```python
from build123d import *

# Parameters (mm, degrees)
BOSS_EXTRUDE1_DEPTH = 1.27
SKETCH2_R           = 21.405
BOSS_EXTRUDE2_DEPTH = 152.4
SKETCH3_R           = 20.5
CUT_EXTRUDE1_DEPTH  = 149.86
SKETCH4_R           = 3
SKETCH4_R_2         = 2
BOSS_EXTRUDE3_DEPTH = 30


with BuildPart() as part:
    # Sketch1 → Boss-Extrude1 (new body)
    with BuildSketch(Plane.XY):
        with BuildLine():
            Line((-7.64, 22.37), (7.64, 22.37))
            ThreePointArc((7.64, 22.37), (30.01, 0), (7.64, -22.37))
            Line((7.64, -22.37), (-7.64, -22.37))
            ThreePointArc((-7.64, -22.37), (-30.01, 0), (-7.64, 22.37))
        make_face()
    extrude(amount=BOSS_EXTRUDE1_DEPTH)

    # Sketch2 → Boss-Extrude2 (add)
    with BuildSketch(Plane.XY.offset(1.27)):
        Circle(SKETCH2_R)
    extrude(amount=BOSS_EXTRUDE2_DEPTH)

    # Sketch3 → Cut-Extrude1 (cut)
    with BuildSketch(Plane(origin=(0, 0, 0), x_dir=(-1, 0, 0), z_dir=(0, 0, -1))):
        Circle(SKETCH3_R)
    extrude(amount=-CUT_EXTRUDE1_DEPTH, mode=Mode.SUBTRACT)

    # Sketch4 → Boss-Extrude3 (add)
    with BuildSketch(Plane.XY.offset(153.67)):
        Circle(SKETCH4_R)
        Circle(SKETCH4_R_2, mode=Mode.SUBTRACT)
    extrude(amount=BOSS_EXTRUDE3_DEPTH)


solid = part.part
```
Read the model definition and answer for the solid it produces. Units are mm, in the model's axes. A direction names the side the tool comes from. Coordinates: 2 decimals unless noted, no trailing zeros. Write each loop counter-clockwise with the first axis right and the second up, starting at its lowest first coordinate (ties: lowest second). Pieces come first, ordered by that corner, then holes. Notation, with made-up numbers: (69, 16.25) -> (109, 16.25) arc R27 cw to (109, 55.25) -> close; hole circle Ø2 at (-10, -24.75). An arc over 180 degrees is marked (long way). Answer as a JSON object with one key per item and string values.
Q1. The part is cut by section D-D on x = 13. Give the vertices of the cut face in (y, z), then the cut area to 3 significant figures.
The answers:
{"outline": "(-21.72, 0) -> (-15.85, 0) -> (-15.85, 149.86) -> (15.85, 149.86) -> (15.85, 0) -> (21.72, 0) -> (21.72, 1.27) -> (17.01, 1.27) -> (17.01, 153.67) -> (-17.01, 153.67) -> (-17.01, 1.27) -> (-21.72, 1.27) -> close", "area": "488 mm2"}
Q2. The part is cut by section C-C on x = 0. Give the vertices of the cut face in (y, z) (3 decimals), then the cut area to 3 significant figures.
The answers:
{"outline": "(-22.37, 0) -> (-20.5, 0) -> (-20.5, 149.86) -> (20.5, 149.86) -> (20.5, 0) -> (22.37, 0) -> (22.37, 1.27) -> (21.405, 1.27) -> (21.405, 153.67) -> (3, 153.67) -> (3, 183.67) -> (2, 183.67) -> (2, 153.67) -> (-2, 153.67) -> (-2, 183.67) -> (-3, 183.67) -> (-3, 153.67) -> (-21.405, 153.67) -> (-21.405, 1.27) -> (-22.37, 1.27) -> close", "area": "497 mm2"}
Q3. The part is cut by section A-A on z = 133. Give the vertices of the cut face in (x, y) (3 decimals).
The answers:
{"outline": "circle Ø42.81 at (0, 0); hole circle Ø41 at (0, 0)"}
Q4. Determine the mould class of faces 1 (the cylindrical face through (4.444, -20.013, 73.881)), 2 (the flat face through (20.1, -4.9, 0)), 3 (the cylindrical face through (30.005, 0.492, 0.626)) for opening direction Y: pulls with the +Y half, pulls with the -Y half, needs draft (parallel to the pull), parting line crosses it, or undercut.
The answers:
{"face 1": "undercut", "face 2": "needs draft", "face 3": "parting line crosses it"}
Q5. A tool of negligible diameter and unlimited length cuts with its end or side. For faces 4 (the flat face through (0, 0, 149.86)), 5 (the flat face through (0, 0, 153.67)), 6 (the cylindrical face through (-30.005, -0.492, 0.626)), from which of +Z, -Z, +X, -X, +Y, -Y can it reach the whole face along a straight path? Write none if from no direction.
The answers:
{"face 4": "-Z", "face 5": "+Z", "face 6": "+Z, -Z, -X"}
Q6. Consider line 1 (Y direction, x = 0, z = 171.5); line 2 (Y direction, x = 0, z = 79) (3 decimals); line 3 (Z direction, x = -14, y = -19). Determine where each line is inside the solid, lowest interval first. Write a range as [from, to].
The answers:
{"line 1": "y = [-3, -2], [2, 3]", "line 2": "y = [-21.405, -20.5], [20.5, 21.405]", "line 3": "z = [0, 1.27]"}
Q7. Flat-ended cylindrical pins translate along their axes: pin 1 Ø5 at (y, z) = (11.5, 138.5) entering from -X; pin 2 Ø6 at (y, z) = (-13.5, 33) entering from +X; pin 3 Ø2 at (x, y) = (-8.5, -10.5) entering from -Z. Find the tip coordinate at first contact, or state that the pin passes through.
The answers:
{"pin 1": "stops at x = -19.42", "pin 2": "stops at x = 18.65", "pin 3": "stops at z = 149.86"}
Q8. The part is cut by section B-B on y = 0. Give the vertices of the cut face in (x, z) (3 decimals), then the cut area to 3 significant figures.
The answers:
{"outline": "(-30.01, 0) -> (-20.5, 0) -> (-20.5, 149.86) -> (20.5, 149.86) -> (20.5, 0) -> (30.01, 0) -> (30.01, 1.27) -> (21.405, 1.27) -> (21.405, 153.67) -> (3, 153.67) -> (3, 183.67) -> (2, 183.67) -> (2, 153.67) -> (-2, 153.67) -> (-2, 183.67) -> (-3, 183.67) -> (-3, 153.67) -> (-21.405, 153.67) -> (-21.405, 1.27) -> (-30.01, 1.27) -> close", "area": "516 mm2"}
